```python
from build123d import *

# Parameters (mm, degrees)
EXTRUDE_1_DEPTH     = 2
SKETCH_3_R          = 1
CUT_EXTRUDE_1_DEPTH = 2
EXTRUDE_2_DEPTH     = 10
CUT_EXTRUDE_2_DEPTH = 20
SKETCH_9_W          = 3
SKETCH_9_H          = 8.464174718
CUT_EXTRUDE_3_DEPTH = 10


with BuildPart() as part:
    # 草图2 → 凸台-拉伸1 (new body)
    with BuildSketch(Plane(origin=(0, 0, 0), x_dir=(1, 0, 0), z_dir=(0, 1, 0))):
        with BuildLine():
            Line((-10.13605196, 2.25), (-1.801845215, 2.25))
            Line((-1.801845215, 2.25), (-1.801845215, 4))
            ThreePointArc((-1.801845215, 4), (0, 5.801845215), (1.801845215, 4))
            Line((1.801845215, 4), (1.801845215, 2.25))
            Line((1.801845215, 2.25), (10.13605196, 2.25))
            ThreePointArc((10.13605196, 2.25), (12.38605196, 0), (10.13605196, -2.25))
            Line((10.13605196, -2.25), (-10.13605196, -2.25))
            ThreePointArc((-10.13605196, -2.25), (-12.38605196, 0), (-10.13605196, 2.25))
        make_face()
    extrude(amount=EXTRUDE_1_DEPTH)

    # 草图3 → 切除-拉伸1 (cut)
    with BuildSketch(Plane(origin=(0, 2, 0), x_dir=(1, 0, 0), z_dir=(0, 1, 0))):
        with Locations(Location((0, 4.027870037, 0), (0, 0, 270))):
            Circle(SKETCH_3_R)
    extrude(amount=-CUT_EXTRUDE_1_DEPTH, mode=Mode.SUBTRACT)

    # 草图4 → 凸台-拉伸2 (add, symmetric)
    with BuildSketch(Plane(origin=(0, 0, 0), x_dir=(0, 0, -1), z_dir=(1, 0, 0))):
        with BuildLine():
            Line((2.25, 2), (0.533443954, 5.615166387))
            ThreePointArc((0.533443954, 5.615166387), (-2.053385242, 6.980617435), (-3.235702378, 4.305123453))
            Line((-3.235702378, 4.305123453), (-2.25, 2))
            Line((-2.25, 2), (2.25, 2))
        make_face()
    extrude(amount=EXTRUDE_2_DEPTH, both=True)

    # 草图8 → 切除-拉伸2 (cut)
    with BuildSketch(Plane.ZY.offset(10)):
        Polygon((0.599367488, 3.232629101), (2.322446911, 3.408689608), (3.031513751, 4.988950414), (2.017501168, 6.393150714), (0.294421745, 6.217090207), (-0.414645095, 4.6368294), align=None)
    extrude(amount=-CUT_EXTRUDE_2_DEPTH, mode=Mode.SUBTRACT)

    # 草图9 → 切除-拉伸3 (cut, symmetric)
    with BuildSketch(Plane.XY):
        with Locations((-4.5, 6.232087359)):
            Rectangle(SKETCH_9_W, SKETCH_9_H)
        with Locations((4.5, 6.232087359)):
            Rectangle(SKETCH_9_W, SKETCH_9_H)
    extrude(amount=CUT_EXTRUDE_3_DEPTH, both=True, mode=Mode.SUBTRACT)


solid = part.part
```
Source: CAD feature listing. Evaluate the final solid. Frame: model axes, mm. A direction names the side the tool comes from. Coordinates: 2 decimals unless noted, no trailing zeros. Loops run counter-clockwise (first coordinate to the right, second up) from the corner with the lowest first, then second, coordinate; pieces in that order, holes last. Notation, with made-up numbers: M -7,29 L -1,29 A32 cw -1,57 Z; hole C 58.25,88.25 d9. An arc over 180 degrees is marked long. Use a Markdown table: item, result. Add a question column.
Q1. First-contact query: pin 1 (1.6 mm diameter, centred on x = -6, y = 1, fed in from -Z); pin 2 (0.9 mm diameter, centred on x = -4, z = -1, fed in from +Y); pin 3 (1.9 mm diameter, centred on y = 1, z = -3.5, fed in from -X). Flat tips, straight axial feed; report the tip coordinate or a pass-through.
Q2. Draft query along Z for faces 4 (the flat face through (-0.042, 5.681, 2.532)), 5 (the flat face through (-11, 2, 0)), 6 (the flat face through (-7.97, 3.17, 2.75)). Return one class per face: pulls with the +Z half, pulls with the -Z half, needs draft (parallel to the pull), parting line crosses it, or undercut.
Q3. Section query C-C, the plane y = 1. Return loops of the section in (x, z), and give its area (3 significant figures).
Q4. Access query for faces 1 (the flat face through (7.972, 6.306, 1.168)), 2 (the flat face through (0.03, 2, -2.87)), 3 (the flat face through (-1.802, 1, -3)). Directions: +Z, -Z, +X, -X, +Y, -Y. A direction counts if a zero-diameter tool reaches every point of the face in a straight line with its end or side. Return the directions, or none.
Q5. Section query A-A, the plane x = 0. Return loops of the section in (y, z), and give its area (3 significant figures).
Q6. Section query B-B, the plane x = -9.5. Return loops of the section in (y, z), and give its area (3 significant figures).
Q7. Material intervals for L1, parallel to X at y = 5.75, z = 0; L2, parallel to Y at x = -5, z = -1.25; L3, parallel to Y at x = 9.75, z = 2.5, sorted ascending.
Q8. Section query D-D, the plane z = -4.75. Return loops of the section in (x, y), and give its area (3 significant figures).
Result:
| question | item | result |
|---|---|---|
| 1 | pin 1 | stops at z = -2.25 |
| 1 | pin 2 | stops at y = 2 |
| 1 | pin 3 | stops at x = -1.8 |
| 2 | face 4 | undercut |
| 2 | face 5 | needs draft |
| 2 | face 6 | pulls with the +Z half |
| 3 | outline | M -10.14,-2.25 L -1.8,-2.25 L -1.8,-4 A1.8 ccw 1.8,-4 L 1.8,-2.25 L 10.14,-2.25 A2.25 ccw 10.14,2.25 L -10.14,2.25 A2.25 ccw Z; hole C 0,-4.03 d2 |
| 3 | area | 115 mm2 |
| 4 | face 1 | +X, -X |
| 4 | face 2 | -Z, +X, -X, +Y |
| 4 | face 3 | -Z, -X, +Y, -Y |
| 5 | outline | M 0,-5.8 L 2,-5.8 L 2,-5.03 L 0,-5.03 Z; M 0,-3.03 L 2,-3.03 L 2,-2.25 L 5.62,-0.53 A2 ccw long 4.31,3.24 L 2,2.25 L 0,2.25 Z; hole M 3.23,0.6 L 4.64,-0.41 L 6.22,0.29 L 6.39,2.02 L 4.99,3.03 L 3.41,2.32 Z |
| 5 | area | 24.3 mm2 |
| 6 | outline | M 0,-2.25 L 2,-2.25 L 5.62,-0.53 A2 ccw long 4.31,3.24 L 2,2.25 L 0,2.25 Z; hole M 3.23,0.6 L 4.64,-0.41 L 6.22,0.29 L 6.39,2.02 L 4.99,3.03 L 3.41,2.32 Z |
| 6 | area | 21.2 mm2 |
| 7 | L1 | x = -10 to -6, -3 to 3, 6 to 10 |
| 7 | L2 | y = 0 to 2 |
| 7 | L3 | y = 2.58 to 3.8, 5.72 to 6.76 |
| 8 | outline | M -1.64,0 L -0.69,0 L -0.69,2 L -1.64,2 Z; M 0.69,0 L 1.64,0 L 1.64,2 L 0.69,2 Z |
| 8 | area | 3.79 mm2 |
